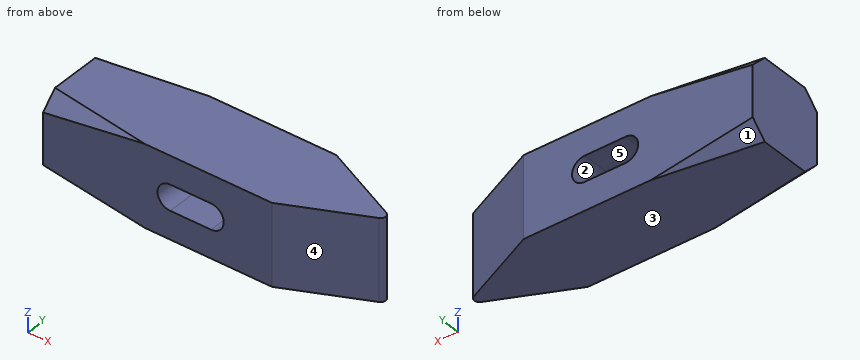
```python
from build123d import *

# Parameters (mm, degrees)
BOSS_EXTRUDE1_DEPTH = 32
CUT_EXTRUDE1_DEPTH  = 32
CUT_EXTRUDE2_DEPTH  = 32
CUT_EXTRUDE3_DEPTH  = 32
CUT_EXTRUDE5_DEPTH  = 32
CUT_EXTRUDE6_DEPTH  = 32


with BuildPart() as part:
    # Sketch1 → Boss-Extrude1 (new body)
    with BuildSketch(Plane.XY):
        with BuildLine():
            Line((0, 16), (0, -16))
            Line((0, -16), (90, -16))
            Line((90, -16), (120.835740498, -1.817013434))
            ThreePointArc((120.835740498, -1.817013434), (122, 0), (120.835740498, 1.817013434))
            Line((120.835740498, 1.817013434), (90, 16))
            Line((90, 16), (0, 16))
        make_face()
    extrude(amount=BOSS_EXTRUDE1_DEPTH)

    # Sketch2 → Cut-Extrude1 (cut)
    with BuildSketch(Plane(origin=(0, 16, 0), x_dir=(1, 0, 0), z_dir=(0, 1, 0))):
        with BuildLine():
            Line((50, -11), (66, -11))
            ThreePointArc((66, -11), (71, -16), (66, -21))
            Line((66, -21), (50, -21))
            ThreePointArc((50, -21), (45, -16), (50, -11))
        make_face()
    extrude(amount=-CUT_EXTRUDE1_DEPTH, mode=Mode.SUBTRACT)

    # Sketch5 → Cut-Extrude2 (cut)
    with BuildSketch(Plane(origin=(-3.114956737, 20.766378245, 20.766378245), x_dir=(0.9944220203272567, 0.07458165152454437, 0.0745816515245444), z_dir=(-0.10547438309019469, 0.70316255393463, 0.70316255393463))):
        Polygon((3.132429364, -7.071067812), (3.132429364, -15.556349186), (43.356800086, -11.313708499), align=None)
    extrude(amount=CUT_EXTRUDE2_DEPTH, mode=Mode.SUBTRACT)

    # Sketch11 → Cut-Extrude3 (cut)
    with BuildSketch(Plane(origin=(-3.114956737, -20.766378245, 20.766378245), x_dir=(0.9944220203272567, -0.07458165152454421, 0.07458165152454423), z_dir=(-0.10547438309019447, -0.7031625539346299, 0.7031625539346302))):
        Polygon((43.356800086, 11.313708499), (3.132429364, 15.556349186), (3.132429364, 7.071067812), align=None)
    extrude(amount=CUT_EXTRUDE3_DEPTH, mode=Mode.SUBTRACT)

    # Sketch12 → Cut-Extrude5 (cut)
    with BuildSketch(Plane(origin=(-0.741656366, -4.944375773, -4.944375773), x_dir=(-0.9944220203272567, 0.07458165152454425, 0.07458165152454425), z_dir=(-0.10547438309019451, -0.70316255393463, -0.70316255393463))):
        Polygon((-40.970187237, -11.313708499), (-0.745816515, -7.071067812), (-0.745816515, -15.556349186), align=None)
    extrude(amount=CUT_EXTRUDE5_DEPTH, mode=Mode.SUBTRACT)

    # Sketch13 → Cut-Extrude6 (cut)
    with BuildSketch(Plane(origin=(-0.741656366, 4.944375773, -4.944375773), x_dir=(0.9944220203272567, 0.07458165152454421, -0.07458165152454421), z_dir=(0.10547438309019444, -0.70316255393463, 0.70316255393463))):
        Polygon((40.970187237, 11.313708499), (0.745816515, 7.071067812), (0.745816515, 15.556349186), align=None)
    extrude(amount=-CUT_EXTRUDE6_DEPTH, mode=Mode.SUBTRACT)


solid = part.part
```
Source: CAD feature listing. Evaluate the final solid. Frame: model axes, mm. Face numbers are marked on the shaded views. A direction names the side the tool comes from. Round coordinates to 2 decimals unless told otherwise and drop trailing zeros. Loops run counter-clockwise (first coordinate to the right, second up) from the corner with the lowest first, then second, coordinate; pieces in that order, holes last.
1. Ray query, L1, parallel to Z at x = 56, y = 13; L2, parallel to X at y = 0, z = 13; L3, parallel to X at y = -1.5, z = 11.5. Return the intervals inside material, ascending.
2. Mould query, pull axis X, two halves, no side actions, for the marked faces 1, 2 and 3. Classes: released by +X, released by -X, zero draft, split by the parting line, or undercut.
3. Section query C-C on y = -6. Output: boundary loops of the cut face in (x, z), and give its area (3 significant figures).
4. Section query D-D on y = 12.5. Output: boundary loops of the cut face in (x, z).
5. Access query for the marked faces 4 and 5. Directions: +Z, -Z, +X, -X, +Y, -Y. A direction counts if a zero-diameter tool reaches every point of the face in a straight line with its end or side. Return the directions, or none.
6. Section query A-A on z = 16. Output: boundary loops of the cut face in (x, y), and give its area (3 significant figures).
7. Contact query for flat-ended pins moving along their axis: pin 1 (1.5 mm diameter, centred on y = 10, z = 6.5, fed in from +X); pin 2 (2 mm diameter, centred on y = -1.5, z = 6, fed in from +X); pin 3 (6 mm diameter, centred on y = 11.5, z = 17.5, fed in from +X). Output: stop coordinate, or through.
8. Section query B-B on x = 47.5. Output: boundary loops of the cut face in (y, z).
Answers below:
1. L1: z = 0 to 11, 21 to 32
1. L2: x = 0 to 46, 70 to 122
1. L3: x = 0 to 47.82, 68.18 to 121.32
2. face 1: released by -X
2. face 2: undercut
2. face 3: zero draft
3. outline: (0, 0) - (111.74, 0) - (111.74, 32) - (0, 32) - close; hole (50, 11) - (66, 11) arc R5 ccw to (66, 21) - (50, 21) arc R5 ccw to start
3. area: 3,340 mm2
4. outline: (0, 2.5) - (16.67, 0) - (97.61, 0) - (97.61, 32) - (16.67, 32) - (0, 29.5) - close; hole (50, 11) - (66, 11) arc R5 ccw to (66, 21) - (50, 21) arc R5 ccw to start
5. face 4: +Z, -Z, +X, -Y
5. face 5: +Y, -Y
6. outline: (0, -16) - (45, -16) - (45, 16) - (0, 16) - close; (71, -16) - (90, -16) - (120.84, -1.82) arc R2 ccw to (120.84, 1.82) - (90, 16) - (71, 16) - close
6. area: 2,600 mm2
7. pin 1: stops at x = 104.68
7. pin 2: stops at x = 121.94
7. pin 3: stops at x = 106.31
8. outline: (-16, 0) - (16, 0) - (16, 11.67) - (-16, 11.67) - close; (-16, 20.33) - (16, 20.33) - (16, 32) - (-16, 32) - close
